Work out the finished part from the listing and answer in its coordinate system (mm). A direction names the side the tool comes from. Coordinates: 2 decimals unless noted, no trailing zeros. Loops run counter-clockwise (first coordinate to the right, second up) from the corner with the lowest first, then second, coordinate; pieces in that order, holes last.
```python
from build123d import *

# Parameters (mm, degrees)
F0_W          = 180
F0_H          = 160
F1_DEPTH      = 1
F2_W          = 10
F2_H          = 10
F3_DEPTH      = 50
F4_T          = 1
F4_T3_DEPTH   = 12
F4_T5_DEPTH   = 12
F4_T7_DEPTH   = 12
F4_T9_DEPTH   = 12
F5_W          = 180
F5_H          = 160
F6_DEPTH      = 3
F7_W          = 180
F7_H          = 160
F7_W_2        = 174
F7_H_2        = 154
F8_DEPTH      = 80
F9_W          = 100
F9_H          = 74
F10_DEPTH     = 120
F11_W         = 94
F11_H         = 68
F12_DEPTH     = 40
F14_T1_DEPTH  = 125
F14_T3_DEPTH  = 99
F14_T5_DEPTH  = 174
F14_T7_DEPTH  = 154
F14_T13_DEPTH = 166.5
F14_T19_DEPTH = 186.5
F14_T28_DEPTH = 166.5
F14_T34_DEPTH = 186.5
F14_T43_DEPTH = 186.5
F14_T49_DEPTH = 166.5
F14_T58_DEPTH = 166.5
F14_T64_DEPTH = 186.5
F15_R         = 6.0326848408
F16_DEPTH     = 500
F17_W         = 180
F17_H         = 160
F18_DEPTH     = 51
F13_W         = 94
F13_H         = 68
F19_DEPTH     = 80


# Not quite as in the source:
# - a fillet or chamfer that OpenCascade refuses, or shapes differently, is made with other operations: its cross-section is extruded or revolved along the edge and cut away or added
# - a shell that OpenCascade refuses in one call is made with other operations: the cavity is built on its own and cut out


with BuildPart() as f1:
    # F0 (on Top) → F1 (new body)
    with BuildSketch(Plane.XY):
        with Locations((-40, 0)):
            Rectangle(F0_W, F0_H)
    extrude(amount=F1_DEPTH)

    # F2 (on face) → F3 (join)
    with BuildSketch(Plane.XY.offset(1)):
        with Locations((-125, 75)):
            Rectangle(F2_W, F2_H)
        with Locations((45, 75)):
            Rectangle(F2_W, F2_H)
        with Locations((-125, -75)):
            Rectangle(F2_W, F2_H)
        with Locations((45, -75)):
            Rectangle(F2_W, F2_H)
    extrude(amount=F3_DEPTH)

    # F4: shell of thickness 1, made by hand


with BuildPart() as f4_core1:
    # F4_t2: copy of F1
    add(f1.part)

    # the walls: a layer under each face that stays
    f4_faces = [f4_core1.faces().sort_by_distance(p)[0] for p in [
        (44, 80, 49.3),
        (-124, -80, 49.3),
        (45, -75, 51),
        (45, -70, 26),
        (40, -75, 26),
        (-120, -75, 26),
        (-125, -70, 26),
        (-125, -75, 51),
        (-130, 74.6666666667, 49.3),
        (-125, 70, 26),
        (-125, 75, 51),
        (-120, 75, 26),
        (-40, 0, 1),
        (45, 70, 26),
        (40, 75, 26),
        (45, 75, 51),
        (50, -74.6666666667, 49.3),
    ]]
    thicken(f4_faces, amount=-F4_T, mode=Mode.SUBTRACT)

    # F4_s4 → F4_t3 (cut)
    with BuildSketch(Plane.YZ.offset(39)):
        Polygon((-69.99, 1.01), (-71, 1), (-71, 0), (-70, 0), align=None)
        Polygon((69.99, 1.01), (70, 0), (71, 0), (71, 1), align=None)
    extrude(amount=F4_T3_DEPTH, mode=Mode.SUBTRACT)

    # F4_s6 → F4_t5 (cut)
    with BuildSketch(Plane.XZ.offset(69)):
        Polygon((39.99, 1.01), (41, 1), (41, 0), (40, 0), align=None)
        Polygon((-119.99, 1.01), (-121, 1), (-121, 0), (-120, 0), align=None)
    extrude(amount=F4_T5_DEPTH, mode=Mode.SUBTRACT)

    # F4_s8 → F4_t7 (cut)
    with BuildSketch(Plane.YZ.offset(-131)):
        Polygon((-69.99, 1.01), (-71, 1), (-71, 0), (-70, 0), align=None)
        Polygon((69.99, 1.01), (71, 1), (71, 0), (70, 0), align=None)
    extrude(amount=F4_T7_DEPTH, mode=Mode.SUBTRACT)

    # F4_s10 → F4_t9 (cut)
    with BuildSketch(Plane.XZ.offset(-81)):
        Polygon((-119.99, 1.01), (-121, 1), (-121, 0), (-120, 0), align=None)
        Polygon((39.99, 1.01), (40, 0), (41, 0), (41, 1), align=None)
    extrude(amount=F4_T9_DEPTH, mode=Mode.SUBTRACT)


with BuildPart() as f1_1:
    add(f1.part)

    # what is left inside the walls is the cavity
    f4_cavity = [f4_core1.part.solids().sort_by_distance(p)[0] for p in [
        (45, 78.99, 33.333333),
        (-125, 78.99, 33.333333),
        (48.99, -75, 33.333333),
        (-123.666667, -71.01, 25),
    ]]
    add(f4_cavity, mode=Mode.SUBTRACT)

    # F5 (on face) → F6 (join)
    with BuildSketch(Plane.XY.offset(51)):
        with Locations((-40, 0)):
            Rectangle(F5_W, F5_H)
    extrude(amount=F6_DEPTH)

    # F7 (on face) → F8 (join)
    with BuildSketch(Plane.XY.offset(54)):
        with Locations((-40, 0)):
            Rectangle(F7_W, F7_H)
        with Locations((-40, 0)):
            Rectangle(F7_W_2, F7_H_2, mode=Mode.SUBTRACT)
    extrude(amount=F8_DEPTH)

    # F9 (on face) → F10 (join)
    with BuildSketch(Plane.XY.offset(54)):
        with Locations((-40, 0)):
            Rectangle(F9_W, F9_H)
    extrude(amount=F10_DEPTH)

    # F11 (on face) → F12 (cut)
    with BuildSketch(Plane.XY.offset(174)):
        with Locations((-40, 0)):
            Rectangle(F11_W, F11_H)
    extrude(amount=-F12_DEPTH, mode=Mode.SUBTRACT)

    # F14: fillet of radius 5 on 8 edges, made by hand

    # F14_s2 → F14_t1 (cut)
    with BuildSketch(Plane.YZ.offset(-102.5)):
        with BuildLine():
            ThreePointArc((-37, 169), (-35.5355339059, 172.5355339059), (-32, 174))
            Line((-32, 174), (-37, 174))
            Line((-37, 174), (-37, 169))
        make_face()
        with BuildLine():
            ThreePointArc((37, 169), (35.5355339059, 172.5355339059), (32, 174))
            Line((32, 174), (37, 174))
            Line((37, 174), (37, 169))
        make_face()
    extrude(amount=F14_T1_DEPTH, mode=Mode.SUBTRACT)

    # F14_s4 → F14_t3 (cut)
    with BuildSketch(Plane.XZ.offset(-49.5)):
        with BuildLine():
            ThreePointArc((-90, 169), (-88.5355339059, 172.5355339059), (-85, 174))
            Line((-85, 174), (-90, 174))
            Line((-90, 174), (-90, 169))
        make_face()
        with BuildLine():
            ThreePointArc((10, 169), (8.5355339059, 172.5355339059), (5, 174))
            Line((5, 174), (10, 174))
            Line((10, 174), (10, 169))
        make_face()
    extrude(amount=F14_T3_DEPTH, mode=Mode.SUBTRACT)

    # F14_s6 → F14_t5 (cut)
    with BuildSketch(Plane.YZ.offset(-127)):
        with BuildLine():
            ThreePointArc((-82, 134), (-78.4644660941, 132.5355339059), (-77, 129))
            Line((-77, 129), (-77, 134))
            Line((-77, 134), (-82, 134))
        make_face()
        with BuildLine():
            ThreePointArc((82, 134), (78.4644660941, 132.5355339059), (77, 129))
            Line((77, 129), (77, 134))
            Line((77, 134), (82, 134))
        make_face()
    extrude(amount=F14_T5_DEPTH, mode=Mode.SUBTRACT)

    # F14_s8 → F14_t7 (cut)
    with BuildSketch(Plane.XZ.offset(-77)):
        with BuildLine():
            ThreePointArc((52, 134), (48.4644660941, 132.5355339059), (47, 129))
            Line((47, 129), (47, 134))
            Line((47, 134), (52, 134))
        make_face()
        with BuildLine():
            ThreePointArc((-132, 134), (-128.4644660941, 132.5355339059), (-127, 129))
            Line((-127, 129), (-127, 134))
            Line((-127, 134), (-132, 134))
        make_face()
    extrude(amount=F14_T7_DEPTH, mode=Mode.SUBTRACT)


with BuildPart() as f14_tool11:
    # F14_s12 → F14_t13 (new body)
    with BuildSketch(Plane.XZ.offset(-77)):
        with BuildLine():
            ThreePointArc((52, 134), (48.4644660941, 132.5355339059), (47, 129))
            Line((47, 129), (47, 134))
            Line((47, 134), (52, 134))
        make_face()
    extrude(amount=F14_T13_DEPTH)

    split(bisect_by=Plane.YZ.offset(50), keep=Keep.BOTTOM)

    split(bisect_by=Plane.XZ.offset(80), keep=Keep.BOTTOM)

    split(bisect_by=Plane.XZ.offset(77), keep=Keep.TOP)


with BuildPart() as f14_tool17:
    # F14_s18 → F14_t19 (new body)
    with BuildSketch(Plane.YZ.offset(59.5)):
        with BuildLine():
            ThreePointArc((-82, 134), (-78.4644660941, 132.5355339059), (-77, 129))
            Line((-77, 129), (-77, 134))
            Line((-77, 134), (-82, 134))
        make_face()
    extrude(amount=-F14_T19_DEPTH)

    split(bisect_by=Plane.YZ.offset(50), keep=Keep.BOTTOM)

    split(bisect_by=Plane.XZ.offset(80), keep=Keep.BOTTOM)

    split(bisect_by=Plane.YZ.offset(47), keep=Keep.TOP)


with BuildPart() as f14_tool11_1:
    add(f14_tool11.part)

    # F14_t23: intersect F14_tool17
    add(f14_tool17.part, mode=Mode.INTERSECT)


with BuildPart() as f1_2:
    add(f1_1.part)

    # F14_t9: cut F14_tool11
    add(f14_tool11_1.part, mode=Mode.SUBTRACT)


with BuildPart() as f14_tool26:
    # F14_s27 → F14_t28 (new body)
    with BuildSketch(Plane.XZ.offset(89.5)):
        with BuildLine():
            ThreePointArc((-132, 134), (-128.4644660941, 132.5355339059), (-127, 129))
            Line((-127, 129), (-127, 134))
            Line((-127, 134), (-132, 134))
        make_face()
    extrude(amount=-F14_T28_DEPTH)

    split(bisect_by=Plane.YZ.offset(-130), keep=Keep.TOP)

    split(bisect_by=Plane.XZ.offset(80), keep=Keep.BOTTOM)

    split(bisect_by=Plane.XZ.offset(77), keep=Keep.TOP)


with BuildPart() as f14_tool32:
    # F14_s33 → F14_t34 (new body)
    with BuildSketch(Plane.YZ.offset(47)):
        with BuildLine():
            ThreePointArc((-82, 134), (-78.4644660941, 132.5355339059), (-77, 129))
            Line((-77, 129), (-77, 134))
            Line((-77, 134), (-82, 134))
        make_face()
    extrude(amount=-F14_T34_DEPTH)

    split(bisect_by=Plane.YZ.offset(-130), keep=Keep.TOP)

    split(bisect_by=Plane.XZ.offset(80), keep=Keep.BOTTOM)

    split(bisect_by=Plane.YZ.offset(-127), keep=Keep.BOTTOM)


with BuildPart() as f14_tool26_1:
    add(f14_tool26.part)

    # F14_t38: intersect F14_tool32
    add(f14_tool32.part, mode=Mode.INTERSECT)


with BuildPart() as f1_3:
    add(f1_2.part)

    # F14_t24: cut F14_tool26
    add(f14_tool26_1.part, mode=Mode.SUBTRACT)


with BuildPart() as f14_tool41:
    # F14_s42 → F14_t43 (new body)
    with BuildSketch(Plane.YZ.offset(-127)):
        with BuildLine():
            ThreePointArc((82, 134), (78.4644660941, 132.5355339059), (77, 129))
            Line((77, 129), (77, 134))
            Line((77, 134), (82, 134))
        make_face()
    extrude(amount=F14_T43_DEPTH)

    split(bisect_by=Plane.XZ.offset(-80), keep=Keep.TOP)

    split(bisect_by=Plane.YZ.offset(50), keep=Keep.BOTTOM)

    split(bisect_by=Plane.YZ.offset(47), keep=Keep.TOP)


with BuildPart() as f14_tool47:
    # F14_s48 → F14_t49 (new body)
    with BuildSketch(Plane.XZ.offset(-89.5)):
        with BuildLine():
            ThreePointArc((52, 134), (48.4644660941, 132.5355339059), (47, 129))
            Line((47, 129), (47, 134))
            Line((47, 134), (52, 134))
        make_face()
    extrude(amount=F14_T49_DEPTH)

    split(bisect_by=Plane.XZ.offset(-80), keep=Keep.TOP)

    split(bisect_by=Plane.YZ.offset(50), keep=Keep.BOTTOM)

    split(bisect_by=Plane.XZ.offset(-77), keep=Keep.BOTTOM)


with BuildPart() as f14_tool41_1:
    add(f14_tool41.part)

    # F14_t53: intersect F14_tool47
    add(f14_tool47.part, mode=Mode.INTERSECT)


with BuildPart() as f1_4:
    add(f1_3.part)

    # F14_t39: cut F14_tool41
    add(f14_tool41_1.part, mode=Mode.SUBTRACT)


with BuildPart() as f14_tool56:
    # F14_s57 → F14_t58 (new body)
    with BuildSketch(Plane.XZ.offset(77)):
        with BuildLine():
            ThreePointArc((-132, 134), (-128.4644660941, 132.5355339059), (-127, 129))
            Line((-127, 129), (-127, 134))
            Line((-127, 134), (-132, 134))
        make_face()
    extrude(amount=-F14_T58_DEPTH)

    split(bisect_by=Plane.XZ.offset(-80), keep=Keep.TOP)

    split(bisect_by=Plane.YZ.offset(-130), keep=Keep.TOP)

    split(bisect_by=Plane.XZ.offset(-77), keep=Keep.BOTTOM)


with BuildPart() as f14_tool62:
    # F14_s63 → F14_t64 (new body)
    with BuildSketch(Plane.YZ.offset(-139.5)):
        with BuildLine():
            ThreePointArc((82, 134), (78.4644660941, 132.5355339059), (77, 129))
            Line((77, 129), (77, 134))
            Line((77, 134), (82, 134))
        make_face()
    extrude(amount=F14_T64_DEPTH)

    split(bisect_by=Plane.XZ.offset(-80), keep=Keep.TOP)

    split(bisect_by=Plane.YZ.offset(-130), keep=Keep.TOP)

    split(bisect_by=Plane.YZ.offset(-127), keep=Keep.BOTTOM)


with BuildPart() as f14_tool56_1:
    add(f14_tool56.part)

    # F14_t68: intersect F14_tool62
    add(f14_tool62.part, mode=Mode.INTERSECT)


with BuildPart() as f1_5:
    add(f1_4.part)

    # F14_t54: cut F14_tool56
    add(f14_tool56_1.part, mode=Mode.SUBTRACT)

    # F15 (on face) → F16 (cut)
    with BuildSketch(Plane.YZ.offset(10)):
        with Locations((0, 173)):
            Circle(F15_R)
    extrude(amount=-F16_DEPTH, mode=Mode.SUBTRACT)

    # F17 (on face) → F18 (cut)
    with BuildSketch(Plane(origin=(0, 0, 0), x_dir=(1, 0, 0), z_dir=(0, 0, -1))):
        with Locations((-40, 0)):
            Rectangle(F17_W, F17_H)
    extrude(amount=-F18_DEPTH, mode=Mode.SUBTRACT)

    # F13 (on face) → F19 (cut)
    with BuildSketch(Plane(origin=(0, 0, 51), x_dir=(1, 0, 0), z_dir=(0, 0, -1))):
        with Locations((-40, 0)):
            Rectangle(F13_W, F13_H)
    extrude(amount=-F19_DEPTH, mode=Mode.SUBTRACT)


solid = f1_5.part
```
1. A cutting plane is placed at B-B, the plane y = 12. Give the vertices of the cut face in (x, z), then the cut area to 3 significant figures.
2. A cutting plane is placed at C-C, the plane x = 33.5. Give the vertices of the cut face in (y, z).
3. Each of these flat-tipped pins is pushed along its axis until it touches: P1, Ø1, axis at x = -63, y = 20, coming from the +Z side; P2, Ø3, axis at x = -25, y = -19, coming from the -Z side; P3, Ø6, axis at x = -60.5, z = 158.5, coming from the -Y side. Where does it stop, or does it pass through?
4. For faces 4 (the flat face through (-41, 34, 90)), 5 (the cylindrical face through (-41, 36, 172)), 6 (the flat face through (47, 1, 92)), determine the directions among +Z, -Z, +X, -X, +Y, -Y from which every point of the face is accessible in a straight line to the end or side of a thin tool.
5. A cutting plane is placed at D-D, the plane x = -43.5. Give the vertices of the cut face in (y, z), then the cut area to 3 significant figures.
6. Straight lines are drawn through the part: probe 1 along X at (y, z) = (-14, 78); probe 2 along X at (y, z) = (17.5, 145); probe 3 along X at (y, z) = (63, 58). For each, find the intervals that lie inside material, in ascending order.
7. Determine the mould class of faces 1 (the flat face through (-41, -80, 92)), 2 (the flat face through (50, -1, 92)), 3 (the flat face through (-127, 1, 92)) for opening direction Y: released by +Y, released by -Y, zero draft, split by the parting line, or undercut.
8. A cutting plane is placed at A-A, the plane z = 81. Give the vertices of the cut face in (x, y).
Answers below:
1. outline: (-130, 51) - (-87, 51) - (-87, 131) - (7, 131) - (7, 51) - (50, 51) - (50, 133.58) arc R5 ccw to (47, 129) - (47, 54) - (10, 54) - (10, 169) arc R5 ccw to (7, 173.58) - (7, 134) - (-87, 134) - (-87, 173.58) arc R5 ccw to (-90, 169) - (-90, 54) - (-127, 54) - (-127, 129) arc R5 ccw to (-130, 133.58) - close
1. area: 1,720 mm2
2. outline: (-80, 51) - (80, 51) - (80, 133.58) arc R5 ccw to (77, 129) - (77, 54) - (-77, 54) - (-77, 129) arc R5 ccw to (-80, 133.58) - close
3. P1: stops at z = 134
3. P2: stops at z = 131
3. P3: stops at y = -37
4. face 4: -Z
4. face 5: +Z, +X, -X, +Y
4. face 6: +Z
5. outline: (-80, 51) - (-34, 51) - (-34, 131) - (34, 131) - (34, 51) - (80, 51) - (80, 133.58) arc R5 ccw to (77, 129) - (77, 54) - (37, 54) - (37, 169) arc R5 ccw to (34, 173.58) - (34, 134) - (-34, 134) - (-34, 173.58) arc R5 ccw to (-37, 169) - (-37, 54) - (-77, 54) - (-77, 129) arc R5 ccw to (-80, 133.58) - close
5. area: 1,660 mm2
6. probe 1: x = -130 to -127, -90 to -87, 7 to 10, 47 to 50
6. probe 2: x = -90 to -87, 7 to 10
6. probe 3: x = -130 to -127, 47 to 50
7. face 1: released by -Y
7. face 2: zero draft
7. face 3: undercut
8. outline: (-130, -80) - (50, -80) - (50, 80) - (-130, 80) - close; (-90, -37) - (10, -37) - (10, 37) - (-90, 37) - close; hole (-127, -77) - (47, -77) - (47, 77) - (-127, 77) - close; hole (-87, -34) - (7, -34) - (7, 34) - (-87, 34) - close
